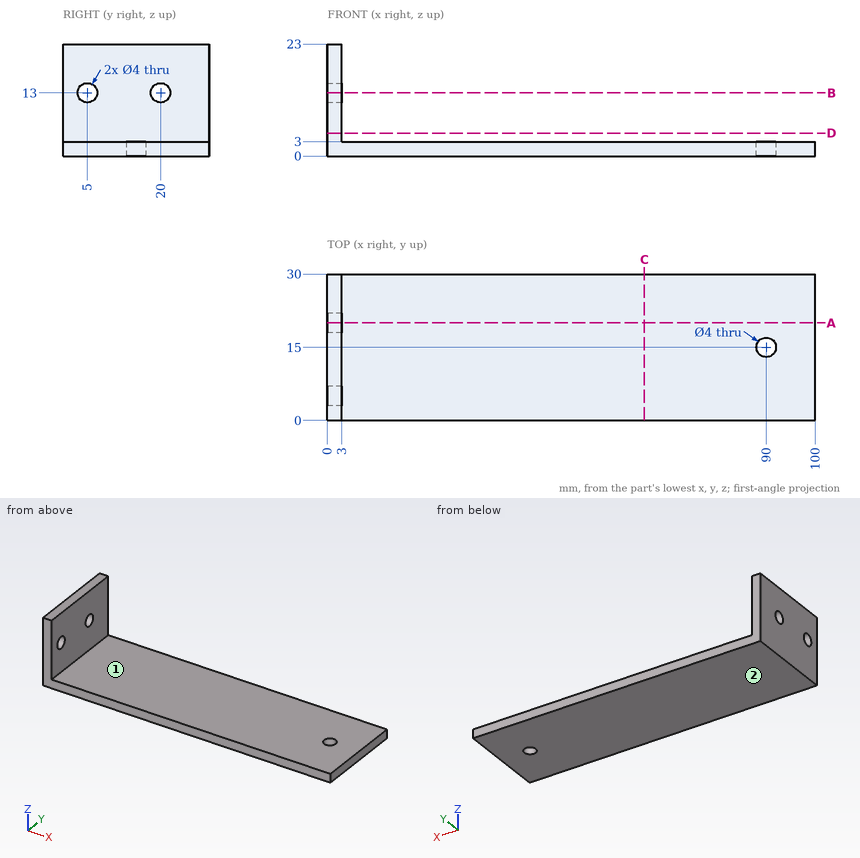
Verification items for this drawing (mm, ordinates from the low corner). A direction names the side the tool comes from. Give positions to 0.01 mm unless a question says otherwise; leave off trailing zeros. Loops run counter-clockwise (first coordinate to the right, second up) from the corner with the lowest first, then second, coordinate; pieces in that order, holes last.
1. Cross-section at B-B on z = 13. Record the cut outline in (x, y).
Derived:
outline: (0, 0) - (3, 0) - (3, 3) - (0, 3) - close; (0, 7) - (3, 7) - (3, 18) - (0, 18) - close; (0, 22) - (3, 22) - (3, 30) - (0, 30) - close
2. Material ranges on probe 1 along Y at (x, z) = (1.9, 13); probe 2 along Y at (x, z) = (90, 1.4); probe 3 along X at (y, z) = (18.5, 15.5), recorded low to high.
Derived:
probe 1: y = 0 to 3, 7 to 18, 22 to 30
probe 2: y = 0 to 13, 17 to 30
probe 3: x = 0 to 3
3. Go/stop test with flat-tipped pins: P1, Ø2, axis at x = 75, y = 27, coming from the +Z side; P2, Ø6.5, axis at y = 20, z = 13, coming from the -X side; P3, Ø6, axis at y = 18.5, z = 17.5, coming from the +X side. Record where each tip stops, or that it passes through.
Derived:
P1: stops at z = 3
P2: stops at x = 0
P3: stops at x = 3
4. Cross-section at A-A on y = 20. Record the cut outline in (x, z), and give its area (3 significant figures).
Derived:
outline: (0, 0) - (100, 0) - (100, 3) - (3, 3) - (3, 11) - (0, 11) - close; (0, 15) - (3, 15) - (3, 23) - (0, 23) - close
area: 348 mm2
5. Cross-section at D-D on z = 4.75. Record the cut outline in (x, y).
Derived:
outline: (0, 0) - (3, 0) - (3, 30) - (0, 30) - close
6. Cross-section at C-C on x = 65. Record the cut outline in (y, z), and give its area (3 significant figures).
Derived:
outline: (0, 0) - (30, 0) - (30, 3) - (0, 3) - close
area: 90.0 mm2
7. Tool access check on the marked faces 1 and 2. Record the directions out of +Z, -Z, +X, -X, +Y, -Y that give a thin tool (end or side, any length) a straight path to the whole face; none if there is none.
Derived:
face 1: +Z, +X, +Y, -Y
face 2: -Z, +X, -X, +Y, -Y
